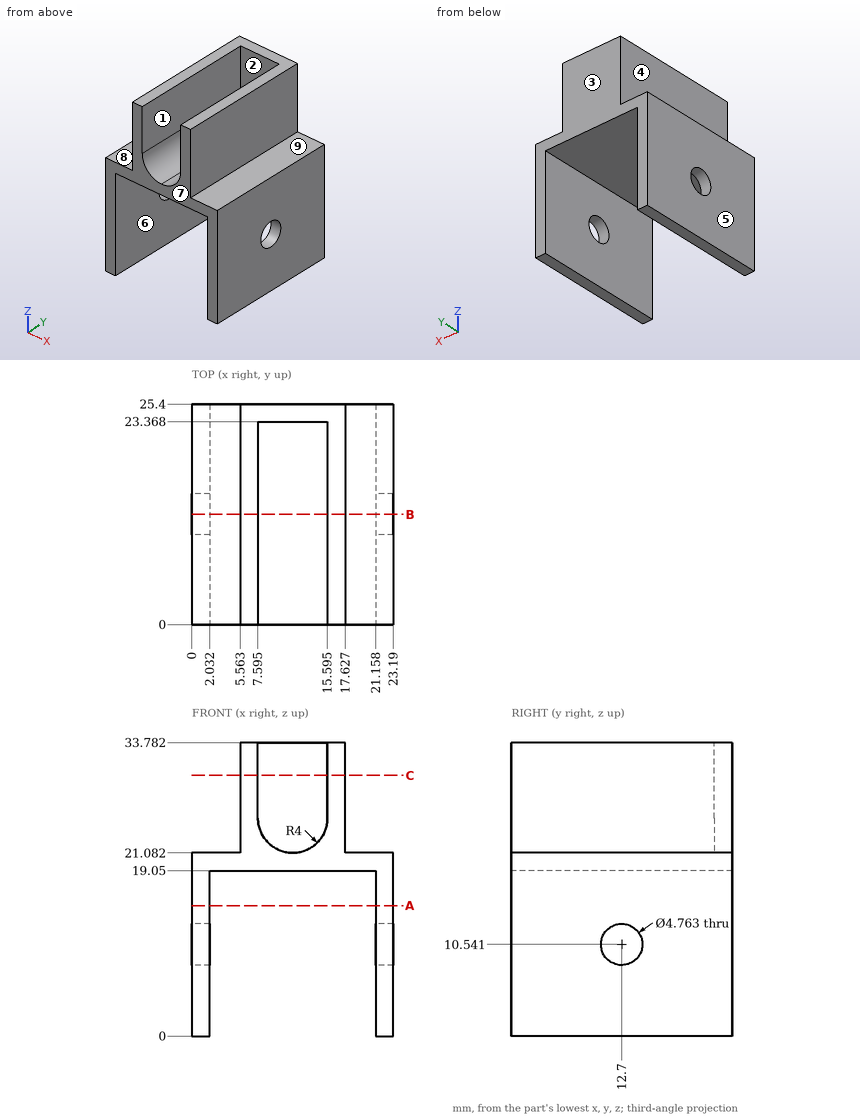
Input: dimensioned drawing with shaded views. Units: mm. Origin: part minimum x, y, z. A direction names the side the tool comes from. Round coordinates to 2 decimals unless told otherwise and drop trailing zeros. Order: outer loops, then holes, each group sorted by start corner. A loop starts at its lowest first (then second) coordinate and runs counter-clockwise, first axis right, second up.
Q1. Mould query, pull axis X, two halves, no side actions, for the marked faces 1, 2, 3 and 4. Classes: released by +X, released by -X, zero draft, split by the parting line, or undercut.
Result sheet:
face 1: undercut
face 2: undercut
face 3: zero draft
face 4: released by -X
Q2. Section C-C, the plane z = 30. Output: boundary loops of the cut face in (x, y) (1 decimal).
Result sheet:
outline: (5.6, 0) - (7.6, 0) - (7.6, 23.4) - (15.6, 23.4) - (15.6, 0) - (17.6, 0) - (17.6, 25.4) - (5.6, 25.4) - close
Q3. Pin query (flat end, axial travel): pin 1 (10 mm diameter, centred on x = 11, y = 11, fed in from +Z); pin 2 (4.5 mm diameter, centred on x = 21, y = 10.5, fed in from +Z); pin 3 (1 mm diameter, centred on x = 13, y = 22.5, fed in from +Z) (1 decimal); pin 4 (4 mm diameter, centred on y = 10, z = 26, fed in from -X). Return the tip coordinate at first contact, or that it passes through.
Result sheet:
pin 1: stops at z = 33.78
pin 2: stops at z = 21.08
pin 3: stops at z = 21.6
pin 4: stops at x = 5.56
Q4. Section A-A, the plane z = 15. Output: boundary loops of the cut face in (x, y).
Result sheet:
outline: (0, 0) - (2.03, 0) - (2.03, 25.4) - (0, 25.4) - close; (21.16, 0) - (23.19, 0) - (23.19, 25.4) - (21.16, 25.4) - close
Q5. Material intervals for probe 1 along X at (y, z) = (11.75, 31) (1 decimal); probe 2 along X at (y, z) = (6.25, 3); probe 3 along Z at (x, y) = (22.35, 12.7), sorted ascending.
Result sheet:
probe 1: x = 5.6 to 7.6, 15.6 to 17.6
probe 2: x = 0 to 2.03, 21.16 to 23.19
probe 3: z = 0 to 8.16, 12.92 to 21.08
Q6. Access query for the marked faces 5, 6, 7, 8 and 9. Directions: +Z, -Z, +X, -X, +Y, -Y. A direction counts if a zero-diameter tool reaches every point of the face in a straight line with its end or side. Return the directions, or none.
Result sheet:
face 5: +Z, -Z, -X, +Y, -Y
face 6: -Z, +Y, -Y
face 7: +Z, -Z, +X, -X, -Y
face 8: +Z, -X, +Y, -Y
face 9: +Z, +X, +Y, -Y
Q7. Section B-B, the plane y = 12.7. Give the number of separate pieces and of enclosed holes in the cut face, and give its area (3 significant figures).
Result sheet:
separate pieces: 3
enclosed holes: 0
area: 164 mm2
